```python
from build123d import *

# Parameters (mm, degrees)
SKETCH_W        = 67
SKETCH_H        = 10
PAD_DEPTH       = 40
SKETCH001_W     = 37
SKETCH001_H     = 10
POCKET_DEPTH    = 30
FILLET_R        = 18.45
SKETCH002_R     = 3
POCKET001_DEPTH = 34
SKETCH003_R     = 1.9
POCKET002_DEPTH = 6
FILLET001_R     = 3
FILLET002_R     = 3


with BuildPart() as part:
    # Sketch → Pad (new body)
    with BuildSketch(Plane.XY):
        Rectangle(SKETCH_W, SKETCH_H)
    extrude(amount=PAD_DEPTH)

    # Sketch001 (on Face5 of Pad) → Pocket (cut)
    with BuildSketch(Plane(origin=(0, 0, 0), x_dir=(1, 0, 0), z_dir=(0, 0, -1))):
        Rectangle(SKETCH001_W, SKETCH001_H)
    extrude(amount=-POCKET_DEPTH, mode=Mode.SUBTRACT)

    # Fillet
    fillet_edges = [part.edges().sort_by_distance(p)[0] for p in [
        (-18.5, 0, 30),
        (18.5, 0, 30),
    ]]
    fillet(fillet_edges, radius=FILLET_R)

    # Sketch002 (on Face4 of Fillet) → Pocket001 (cut)
    with BuildSketch(Plane(origin=(0, 0, 0), x_dir=(1, 0, 0), z_dir=(0, 0, -1))):
        with Locations((-10, 0)):
            Circle(SKETCH002_R)
        with Locations((10, 0)):
            Circle(SKETCH002_R)
    extrude(amount=-POCKET001_DEPTH, mode=Mode.SUBTRACT)

    # Sketch003 (on Face8 of Pocket001) → Pocket002 (cut)
    with BuildSketch(Plane.XY.offset(40)):
        with Locations((-10, 0)):
            Circle(SKETCH003_R)
        with Locations((10, 0)):
            Circle(SKETCH003_R)
    extrude(amount=-POCKET002_DEPTH, mode=Mode.SUBTRACT)

    # Fillet001
    fillet001_edges = [part.edges().sort_by_distance(p)[0] for p in [
        (18.5, -5, 5.775),
    ]]
    fillet(fillet001_edges, radius=FILLET001_R)

    # Fillet002
    fillet002_edges = [part.edges().sort_by_distance(p)[0] for p in [
        (-18.5, 5, 5.775),
    ]]
    fillet(fillet002_edges, radius=FILLET002_R)


solid = part.part
```
The model under review builds one solid part; all positions refer to its coordinate system, in mm. A direction names the side the tool comes from. Coordinates: 2 decimals unless noted, no trailing zeros. Order: outer loops, then holes, each group sorted by start corner. A loop starts at its lowest first (then second) coordinate and runs counter-clockwise, first axis right, second up. Notation, with made-up numbers: (70, 60.5) -> (118, 60.5) arc R18 cw to (118, 93.5) -> close; hole circle Ø7 at (-36, -32.75). An arc over 180 degrees is marked (long way). Answer in a Markdown table with one row per item. Add a question column.
Item 1: We need section A-A on y = -1. Write out the cut boundary in (x, z), plus the area to 3 significant figures.
Item 2: Mouldability with a two-part tool opening along Y and no side actions: class faces 1 (the flat face through (33.5, 0, 20)), 2 (the cylindrical face through (12.77, 1.15, 30.31)), 3 (the cylindrical face through (19.4, -4.14, 5.86)) as +Y half, -Y half, draft (parallel to the pull), parting line (faces both ways), or undercut.
Item 3: Clearance check with flat-ended pins moving along their axes: pin 1 (5 mm diameter, centred on x = -11.5, y = -1.5, fed in from -Z); pin 2 (1.5 mm diameter, centred on x = 12.5, y = 2, fed in from -Z); pin 3 (5 mm diameter, centred on x = -10, y = 0, fed in from -Z). State where each tip first meets the part, or that it passes through.
Item 4: Machinability: for faces 4 (the cylindrical face through (3.944, -0.028, 29.584)), 5 (the cylindrical face through (-19.36, 4.1, 5.86)), 6 (the cylindrical face through (-19.4, -4.14, 5.69)), 7 (the flat face through (-8, 1, 34)), which of the approach directions +Z, -Z, +X, -X, +Y, -Y give a long, thin tool a straight path to every point of the face, cutting with its end or side? Answer none if there is none.
Item 5: To check wall thickness, follow probe 1 along X at (y, z) = (0, 27); probe 2 along Y at (x, z) = (10, 37); probe 3 along X at (y, z) = (-2, 21). State the ranges of each line that lie inside material, in increasing order.
Final values:
| question | item | result |
|---|---|---|
| 1 | outline | (-33.5, 0) -> (-18.5, 0) -> (-18.5, 11.55) arc R18.45 cw to (-12.83, 24.86) -> (-12.83, 34) -> (-11.62, 34) -> (-11.62, 40) -> (-33.5, 40) -> close; (-8.38, 34) -> (-7.17, 34) -> (-7.17, 28.57) arc R18.45 cw to (-0.05, 30) -> (0.05, 30) arc R18.45 cw to (7.17, 28.57) -> (7.17, 34) -> (8.38, 34) -> (8.38, 40) -> (-8.38, 40) -> close; (11.62, 34) -> (12.83, 34) -> (12.83, 24.86) arc R18.45 cw to (18.5, 11.55) -> (18.5, 0) -> (33.5, 0) -> (33.5, 40) -> (11.62, 40) -> close |
| 1 | area | 1,600 mm2 |
| 2 | face 1 | draft |
| 2 | face 2 | undercut |
| 2 | face 3 | -Y half |
| 3 | pin 1 | stops at z = 23.62 |
| 3 | pin 2 | stops at z = 24.44 |
| 3 | pin 3 | stops at z = 34 |
| 4 | face 4 | -Z, +Y, -Y |
| 4 | face 5 | -Z, +Y |
| 4 | face 6 | -Z, -Y |
| 4 | face 7 | -Z |
| 5 | probe 1 | x = -33.5 to -13, 13 to 33.5 |
| 5 | probe 2 | y = -5 to -1.9, 1.9 to 5 |
| 5 | probe 3 | x = -33.5 to -15.9, 15.9 to 33.5 |
